Geometry: final body of the model. Coordinates: model frame, mm. A direction names the side the tool comes from. Round coordinates to 2 decimals unless told otherwise and drop trailing zeros. Write each loop counter-clockwise with the first axis right and the second up, starting at its lowest first coordinate (ties: lowest second). Pieces come first, ordered by that corner, then holes. Notation, with made-up numbers: M 67.5,60 L 86.5,60 A25 ccw 86.5,72 Z; hole C 45.25,69.5 d8. An arc over 180 degrees is marked long. Put each result on its own line as item: value. Start each with the question number.
```python
from build123d import *

# Parameters (mm, degrees)
SKETCH_1_R               = 25
EXTRUDE_1_DEPTH          = 8
SKETCH_2_R               = 22.4
CUT_EXTRUDE_1_DEPTH      = 5.6
SKETCH_3_R               = 18.4
CUT_EXTRUDE_2_DEPTH      = 12.5
EXTRUDE_2_DEPTH          = 8
FILLET_1_R               = 8
CUT_EXTRUDE_START        = -15
SKETCH_5_R               = 1.5
CUT_EXTRUDE_3_DEPTH      = 15
FILLET_2_R               = 2
SKETCH_6_R               = 3.5
CUT_EXTRUDE_4_DEPTH      = 2
PATTERN_CIRCULAR_1_COUNT = 4


with BuildPart() as part:
    # 草图1 → 凸台-拉伸1 (new body)
    with BuildSketch(Plane(origin=(0, 0, 0), x_dir=(1, 0, 0), z_dir=(0, 1, 0))):
        with Locations(Location((0, 0, 0), (0, 0, 270))):
            Circle(SKETCH_1_R)
    extrude(amount=EXTRUDE_1_DEPTH)

    # 草图2 → 切除-拉伸1 (cut)
    with BuildSketch(Plane(origin=(0, 8, 0), x_dir=(1, 0, 0), z_dir=(0, 1, 0))):
        with Locations(Location((0, 0, 0), (0, 0, 270))):
            Circle(SKETCH_2_R)
    extrude(amount=-CUT_EXTRUDE_1_DEPTH, mode=Mode.SUBTRACT)

    # 草图3 → 切除-拉伸2 (cut)
    with BuildSketch(Plane(origin=(0, 2.4, 0), x_dir=(1, 0, 0), z_dir=(0, 1, 0))):
        with Locations(Location((0, 0, 0), (0, 0, 270))):
            Circle(SKETCH_3_R)
    extrude(amount=-CUT_EXTRUDE_2_DEPTH, mode=Mode.SUBTRACT)

    # 草图4 → 凸台-拉伸2 (add)
    with BuildSketch(Plane(origin=(0, 0, 0), x_dir=(1, 0, 0), z_dir=(0, 1, 0))):
        with BuildLine():
            Line((0, 25), (-25, 25))
            Line((-25, 25), (-25, 2.6e-08))
            ThreePointArc((-25, 2.6e-08), (-23.301207713, 9.058350794), (-18.435702489, 16.885641052))
            ThreePointArc((-18.435702489, 16.885641052), (-19.445436483, 19.445436483), (-16.885641052, 18.435702489))
            ThreePointArc((-16.885641052, 18.435702489), (-9.058350782, 23.301207718), (0, 25))
        make_face()
        with BuildLine():
            Line((25, 25), (0, 25))
            ThreePointArc((0, 25), (9.210354363, 23.241544108), (17.125028574, 18.213549801))
            ThreePointArc((17.125028574, 18.213549801), (19.682469279, 19.438809921), (18.425448396, 16.896829626))
            ThreePointArc((18.425448396, 16.896829626), (23.298457137, 9.065423048), (25, 0))
            Line((25, 0), (25, 25))
        make_face()
        with BuildLine():
            ThreePointArc((-18.213549801, -17.125028574), (-23.241544113, -9.210354351), (-25, 2.6e-08))
            Line((-25, 2.6e-08), (-25, -25))
            Line((-25, -25), (-5.8e-08, -25))
            ThreePointArc((-5.8e-08, -25), (-9.065423076, -23.298457126), (-16.896829626, -18.425448396))
            ThreePointArc((-16.896829626, -18.425448396), (-19.438809921, -19.682469279), (-18.213549801, -17.125028574))
        make_face()
        with BuildLine():
            Line((25, -25), (25, 0))
            ThreePointArc((25, 0), (23.22561674, -9.250444694), (18.154341838, -17.18778265))
            ThreePointArc((18.154341838, -17.18778265), (19.675883861, -19.675883861), (17.18778265, -18.154341838))
            ThreePointArc((17.18778265, -18.154341838), (9.250444666, -23.225616751), (-5.8e-08, -25))
            Line((-5.8e-08, -25), (25, -25))
        make_face()
    extrude(amount=EXTRUDE_2_DEPTH)

    # 圆角1
    fillet_1_edges = [part.edges().sort_by_distance(p)[0] for p in [
        (-25, 4, -25),
        (25, 4, -25),
        (-25, 4, 25),
        (25, 4, 25),
    ]]
    fillet(fillet_1_edges, radius=FILLET_1_R)

    # 草图5 → 切除-拉伸3 (cut)
    with BuildSketch(Plane(origin=(0, 8, 0), x_dir=(1, 0, 0), z_dir=(0, 1, 0)).offset(CUT_EXTRUDE_START)):
        with Locations(Location((-18.384776311, 18.384776311, 0), (0, 0, 270))):
            Circle(SKETCH_5_R)
        with Locations(Location((18.615223689, 18.384776311, 0), (0, 0, 270))):
            Circle(SKETCH_5_R)
        with Locations(Location((18.615223689, -18.615223689, 0), (0, 0, 270))):
            Circle(SKETCH_5_R)
        with Locations(Location((-18.384776311, -18.615223689, 0), (0, 0, 270))):
            Circle(SKETCH_5_R)
    extrude(amount=CUT_EXTRUDE_3_DEPTH, mode=Mode.SUBTRACT)

    # 圆角2
    fillet_2_edges = [part.edges().sort_by_distance(p)[0] for p in [
        (0, 8, -22.4),
    ]]
    fillet(fillet_2_edges, radius=FILLET_2_R)

    # 草图6 → 切除-拉伸4 (cut)
    with BuildSketch(Plane.XZ):
        with Locations(Location((-18.384776311, 18.615223689, 0), (0, 0, 270))):
            Circle(SKETCH_6_R)
    cut_extrude_4 = extrude(amount=-CUT_EXTRUDE_4_DEPTH, mode=Mode.SUBTRACT)

    # 阵列(圆周)1: 切除-拉伸4 ×4 about axis
    pattern_circular_1_axis = Axis((0, 0, 0), (0, 1, 0))
    for i in range(1, PATTERN_CIRCULAR_1_COUNT):
        add(cut_extrude_4.rotate(pattern_circular_1_axis, i * 360 / PATTERN_CIRCULAR_1_COUNT), mode=Mode.SUBTRACT)


solid = part.part
```
1) Section B-B, the plane z = 0. Output: boundary loops of the cut face in (x, y).
2) Ray query, probe 1 along X at (y, z) = (1.5, -19.5); probe 2 along Y at (x, z) = (16, 10); probe 3 along Z at (x, y) = (-8.5, 1.5). Return the intervals inside material, ascending.
3) Section D-D, the plane z = 19. Give the number of separate pieces and of enclosed holes in the cut face, and give its area (3 significant figures).
4) Draft query along X for faces 1 (the face through (0, 4, 25)), 2 (the face through (0.98, 4.23, -22.38)), 3 (the face through (22.594, 4.056, -22.719)). Return one class per face: +X half, -X half, draft (parallel to the pull), parting line (faces both ways), or undercut.
5) Access query for faces 4 (the face through (21.802, 0.986, -19.374)), 5 (the face through (18.4, 2.4, -3.4)), 6 (the face through (-11, 0, -17)). Directions: +Z, -Z, +X, -X, +Y, -Y. A direction counts if a zero-diameter tool reaches every point of the face in a straight line with its end or side. Return the directions, or none.
6) First-contact query: pin 1 (2 mm diameter, centred on x = 18, z = 17.5, fed in from -Y). Flat tip, straight axial feed; report the tip coordinate or a pass-through.
7) Section A-A, the plane x = 0. Output: boundary loops of the cut face in (y, z), and give its area (3 significant figures).
8) Section C-C, the plane y = 4. Output: boundary loops of the cut face in (x, z), and give its area (3 significant figures).
Solved:
1. outline: M -25,0 L -18.4,0 L -18.4,2.4 L -22.4,2.4 L -22.4,6 A2 ccw -24.4,8 L -25,8 Z; M 18.4,0 L 25,0 L 25,8 L 24.4,8 A2 ccw 22.4,6 L 22.4,2.4 L 18.4,2.4 Z
2. probe 1: x = -24.6 to -21.93, -15.3 to 15, 21.77 to 24.6
2. probe 2: y = 0 to 2.4
2. probe 3: z = -25 to -16.32, 16.32 to 25
3. separate pieces: 3
3. enclosed holes: 0
3. area: 197 mm2
4. face 1: draft
4. face 2: undercut
4. face 3: +X half
5. face 4: -Y
5. face 5: +Y
5. face 6: +Z, -Z, +X, -X, -Y
6. pin 1: stops at y = 2
7. outline: M 0,-25 L 8,-25 L 8,-24.4 A2 ccw 6,-22.4 L 2.4,-22.4 L 2.4,-18.4 L 0,-18.4 Z; M 0,18.4 L 2.4,18.4 L 2.4,22.4 L 6,22.4 A2 ccw 8,24.4 L 8,25 L 0,25 Z
7. area: 59.1 mm2
8. outline: M -25,-17 A8 ccw -17,-25 L 17,-25 A8 ccw 25,-17 L 25,17 A8 ccw 17,25 L -17,25 A8 ccw -25,17 Z; hole C 0,0 d44.8; hole C -18.38,-18.38 d3; hole C -18.38,18.62 d3; hole C 18.62,-18.38 d3; hole C 18.62,18.62 d3
8. area: 840 mm2
